The model under review builds one solid part; all positions refer to its coordinate system, in mm. A direction names the side the tool comes from. Round coordinates to 2 decimals unless told otherwise and drop trailing zeros. Order: outer loops, then holes, each group sorted by start corner. A loop starts at its lowest first (then second) coordinate and runs counter-clockwise, first axis right, second up. Notation, with made-up numbers: M 19,0 L 42,0 A9 ccw 42,6 Z; hole C 88,9.5 d9. An arc over 180 degrees is marked long. Answer as CSV lines item,"result". Start each with the question number.
from build123d import *

# Parameters (mm, degrees)
SKETCH1_W           = 18
SKETCH1_H           = 30
BOSS_EXTRUDE1_DEPTH = 9
SKETCH2_R           = 5.25
CUT_EXTRUDE1_DEPTH  = 6
SKETCH4_R           = 2.75
CUT_EXTRUDE3_DEPTH  = 28
CUT_EXTRUDE4_REACH  = 38.125
SKETCH5_W           = 8.2
SKETCH5_H           = 5.3
CHAMFER3_SIZE       = 5
SKETCH6_R           = 2.95
BOSS_EXTRUDE2_DEPTH = 5
CHAMFER4_SIZE       = 5
CHAMFER4_SIZE2      = 10.722534603


with BuildPart() as part:
    # Sketch1 → Boss-Extrude1 (new, symmetric)
    with BuildSketch(Plane.XY):
        with Locations((-5, -15)):
            Rectangle(SKETCH1_W, SKETCH1_H)
    extrude(amount=BOSS_EXTRUDE1_DEPTH, both=True)

    # Sketch2 → Cut-Extrude1 (cut)
    with BuildSketch(Plane.XZ.offset(30)):
        with Locations((-5, 0)):
            Circle(SKETCH2_R)
    extrude(amount=-CUT_EXTRUDE1_DEPTH, mode=Mode.SUBTRACT)

    # Sketch4 → Cut-Extrude3 (cut)
    with BuildSketch(Plane.XZ.offset(30)):
        with Locations((-5, 0)):
            Circle(SKETCH4_R)
    extrude(amount=-CUT_EXTRUDE3_DEPTH, mode=Mode.SUBTRACT)

    # Sketch5 → Cut-Extrude4 (cut, up to next)
    with BuildSketch(Plane(origin=(4, 0, 0), x_dir=(0, 0, -1), z_dir=(1, 0, 0)), mode=Mode.PRIVATE) as cut_extrude4_sk1:
        with Locations((0, -16.65)):
            Rectangle(SKETCH5_W, SKETCH5_H)
    cut_extrude4_tool1 = extrude(cut_extrude4_sk1.sketch, amount=-CUT_EXTRUDE4_REACH, mode=Mode.PRIVATE) & part.part
    add(cut_extrude4_tool1.solids().sort_by_distance((4, -16.65, 0))[0], mode=Mode.SUBTRACT)

    # Chamfer3
    # the kernel refuses this chamfer: 5 mm, written as the material it takes off along each edge
    with BuildSketch(Plane(origin=(-14, -42.85841494, 9), x_dir=(0.9996219169112968, 0, 0.027495876610586317), z_dir=(0, 1, 0)), Plane(origin=(4, 12.85841494, -9), x_dir=(0.027495876610586317, 0, 0.9996219169112968), z_dir=(0, -1, 0))) as chamfer3_piece_1:
        Polygon((CHAMFER3_SIZE * 0.999621916911, CHAMFER3_SIZE * 0.0274958766106), (-CHAMFER3_SIZE * 0.0274958766106, CHAMFER3_SIZE * 0.999621916911), (0, 0), align=None)
    extrude(amount=55.71682988, mode=Mode.SUBTRACT)
    with BuildSketch(Plane(origin=(-14, -42.85841494, -9), x_dir=(0.9996219169112968, 0, -0.027495876610586317), z_dir=(0, 1, 0)), Plane(origin=(4, 12.85841494, 9), x_dir=(0.027495876610586317, 0, -0.9996219169112968), z_dir=(0, -1, 0))) as chamfer3_piece_2:
        Polygon((CHAMFER3_SIZE * 0.999621916911, -CHAMFER3_SIZE * 0.0274958766106), (-CHAMFER3_SIZE * 0.0274958766106, -CHAMFER3_SIZE * 0.999621916911), (0, 0), align=None)
    extrude(amount=55.71682988, mode=Mode.SUBTRACT)

    # Sketch6 → Boss-Extrude2 (add)
    with BuildSketch(Plane.XZ.offset(30)):
        Polygon((-1, -9), (11, -9), (11, 9), (-1, 9), (4, 4), (4, -4), align=None)
        with Locations((7, 0)):
            Circle(SKETCH6_R, mode=Mode.SUBTRACT)
    extrude(amount=-BOSS_EXTRUDE2_DEPTH)

    # Chamfer4
    chamfer4_edges = [part.edges().sort_by_distance(p)[0] for p in [
        (11, -27.5, 9),
        (11, -27.5, -9),
    ]]
    chamfer4_side = [part.faces().sort_by_distance(p)[0] for p in [
        (11, -27.5, 0),
    ]]
    chamfer(chamfer4_edges, length=CHAMFER4_SIZE, length2=CHAMFER4_SIZE2, reference=chamfer4_side[0])


solid = part.part
Item 1: Consider section A-A (y = -27.25). State the section outline as (x, z) points, and give its area (3 significant figures).
Item 2: For pin 1 (1 mm diameter, centred on x = -1.5, z = -6, fed in from +Y); pin 2 (5 mm diameter, centred on x = -2.5, z = 1, fed in from -Y); pin 3 (2 mm diameter, centred on x = 4, y = -6, fed in from +Z); pin 4 (5 mm diameter, centred on y = -20, z = 0, fed in from +X), all flat-tipped, find the tip position at first contact; note any pin that passes through.
Item 3: Wall thickness on probe 1 along Z at (x, y) = (-5, -6.75); probe 2 along Y at (x, z) = (-3.25, 3); probe 3 along Y at (x, z) = (-10, -1.75): over which ranges is each line inside the solid? List them lowest first. Write a range as [from, to].
Item 4: Consider section C-C (x = -11.25). State the section outline as (y, z) points, and give its area (3 significant figures).
Item 5: Tool access review of faces 4 (the flat face through (2, -12, 6)), 5 (the flat face through (-5, -14, 3)), 6 (the flat face through (5, -25, -3)), 7 (the flat face through (4, -22, 0)): name each direction out of +Z, -Z, +X, -X, +Y, -Y from which nothing blocks a thin tool from reaching the whole face with its end or side.
Item 6: Consider section B-B (z = 0). State the section outline as (x, y) points.
Item 7: Consider section D-D (y = -12). State the section outline as (x, z) points, and give its area (3 significant figures).
Item 8: The part is to be moulded in two halves that separate along Y. For faces 1 (the flat face through (1, -30, 0)), 2 (the flat face through (-4, -15, 9)), 3 (the flat face through (-5, -17, 4.1)), say which applies: +Y half, -Y half, draft (parallel to the pull), parting line (faces both ways), or undercut.
Reported:
1,outline,"M -14,-4 L -9,-9 L 0.28,-9 L 11,-4 L 11,4 L 0.28,9 L -9,9 L -14,4 Z; hole C -5,0 d10.5; hole C 7,0 d5.9"
1,area,"257 mm²"
2,pin 1,"stops at y = 0"
2,pin 2,"stops at y = -24"
2,pin 3,"stops at z = 5"
2,pin 4,"stops at x = 4"
3,probe 1,"z = [-9, -2.75], [2.75, 9]"
3,probe 2,"y = [-24, -19.3], [-14, 0]"
3,probe 3,"y = [-30, -19.3], [-14, 0]"
4,outline,"M -30,-6.75 L 0,-6.75 L 0,6.75 L -30,6.75 Z; hole M -19.3,-4.1 L -14,-4.1 L -14,4.1 L -19.3,4.1 Z"
4,area,"362 mm²"
5,face 4,"+Z, +X, +Y"
5,face 5,"+X, -X"
5,face 6,"+X, +Y"
5,face 7,"+Z, -Z, +X, +Y"
6,outline,"M -14,-30 L -10.25,-30 L -10.25,-24 L -7.75,-24 L -7.75,-19.3 L -14,-19.3 Z; M -14,-14 L -7.75,-14 L -7.75,-2 L -2.25,-2 L -2.25,-14 L 4,-14 L 4,0 L -14,0 Z; M -2.25,-24 L 0.25,-24 L 0.25,-30 L 4.05,-30 L 4.05,-25 L 4,-25 L 4,-19.3 L -2.25,-19.3 Z; M 9.95,-30 L 11,-30 L 11,-25 L 9.95,-25 Z"
7,outline,"M -14,-4 L -9,-9 L -1,-9 L 4,-4 L 4,4 L -1,9 L -9,9 L -14,4 Z; hole C -5,0 d5.5"
7,area,"250 mm²"
8,face 1,"-Y half"
8,face 2,"draft"
8,face 3,"undercut"
